Model file for the job. Use its own axes, mm. Face numbers are marked on the shaded views. A direction names the side the tool comes from. Round coordinates to 2 decimals unless told otherwise and drop trailing zeros. Loops run counter-clockwise (first coordinate to the right, second up) from the corner with the lowest first, then second, coordinate; pieces in that order, holes last. Notation, with made-up numbers: M -35.75,58 L 3.25,58 A16 cw 3.25,69 Z; hole C -25.5,24.5 d7. An arc over 180 degrees is marked long. Use a Markdown table: item, result. Add a question column.
Item 1: Wall check: L1, parallel to Y at x = 0.3, z = 15; L2, parallel to X at y = 50, z = 26.5; L3, parallel to Y at x = 11, z = 23.5. Give the ranges that are in metal, low to high. Write a range as from..to.
Item 2: Saw through at B-B on y = 40.5. Write the cut outline in (x, z).
Item 3: Pin check, flat tips, straight feed: P1, Ø2, axis at x = 1, y = 47, coming from the -Z side; P2, Ø12.5, axis at x = -11, z = 20.5, coming from the +Y side; P3, Ø9, axis at y = 36.5, z = 20.5, coming from the +X side; P4, Ø4, axis at x = -6.5, y = 9.5, coming from the +Z side. Stop position of each tip, or through.
Item 4: Saw through at D-D on y = 9. Write the cut outline in (x, z).
Item 5: Tool access for the marked faces 1 and 2: list every direction of +Z, -Z, +X, -X, +Y, -Y with a clear straight run to the whole face (end or side of a thin tool).
Item 6: Saw through at C-C on x = -0.5. Write the cut outline in (y, z).
Item 7: Two-plate mould, pull along Y, no slides. Class the marked faces 3, 4, 5 and 6: +Y half, -Y half, draft (parallel to the pull), parting line (faces both ways), or undercut.
Item 8: Saw through at A-A on z = 15. Write the cut outline in (x, y), then the cut area to 3 significant figures.
```python
from build123d import *

# Parameters (mm, degrees)
BOSS_EXTRUDE1_DEPTH = 30
SKETCH2_R           = 9.5
CUT_EXTRUDE1_DEPTH  = 70


with BuildPart() as part:
    # Sketch1 → Boss-Extrude1 (new body)
    with BuildSketch(Plane.XY):
        with BuildLine():
            Line((3.75, 0), (15, 0))
            Line((15, 0), (15, -4))
            Line((15, -4), (-15, -4))
            Line((-15, -4), (-15, 0))
            Line((-15, 0), (-3.75, 0))
            ThreePointArc((-3.75, 0), (-3.042893219, 0.292893219), (-2.75, 1))
            Line((-2.75, 1), (-2.75, 61))
            Line((-2.75, 61), (2.75, 61))
            Line((2.75, 61), (2.75, 1))
            ThreePointArc((2.75, 1), (3.042893219, 0.292893219), (3.75, 0))
        make_face()
    extrude(amount=BOSS_EXTRUDE1_DEPTH)

    # Sketch2 → Cut-Extrude1 (cut)
    with BuildSketch(Plane.ZY.offset(2.75)):
        with Locations((15, 40.5)):
            Circle(SKETCH2_R)
    extrude(amount=-CUT_EXTRUDE1_DEPTH, mode=Mode.SUBTRACT)


solid = part.part
```
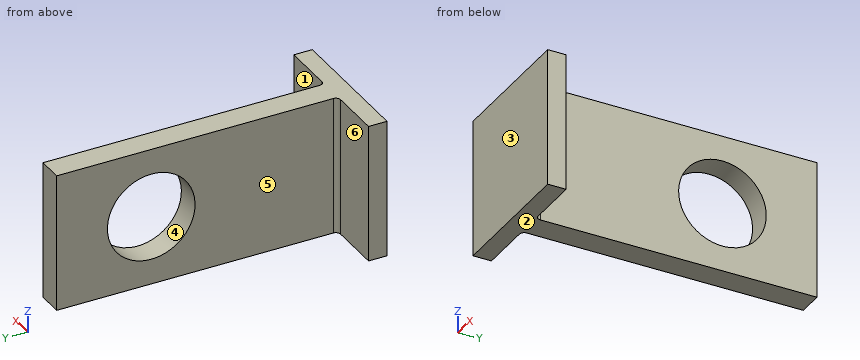
Entries:
| question | item | result |
|---|---|---|
| 1 | L1 | -4..31, 50..61 |
| 1 | L2 | -2.75..2.75 |
| 1 | L3 | -4..0 |
| 2 | outline | M -2.75,0 L 2.75,0 L 2.75,5.5 L -2.75,5.5 Z; M -2.75,24.5 L 2.75,24.5 L 2.75,30 L -2.75,30 Z |
| 3 | P1 | z = 0 |
| 3 | P2 | y = 0 |
| 3 | P3 | x = 2.75 |
| 3 | P4 | through |
| 4 | outline | M -2.75,0 L 2.75,0 L 2.75,30 L -2.75,30 Z |
| 5 | face 1 | +Z, -Z, +X, +Y |
| 5 | face 2 | -Z, +X, -X, +Y, -Y |
| 6 | outline | M -4,0 L 61,0 L 61,30 L -4,30 Z; hole C 40.5,15 d19 |
| 7 | face 3 | -Y half |
| 7 | face 4 | undercut |
| 7 | face 5 | draft |
| 7 | face 6 | +Y half |
| 8 | outline | M -15,-4 L 15,-4 L 15,0 L 3.75,0 A1 cw 2.75,1 L 2.75,31 L -2.75,31 L -2.75,1 A1 cw -3.75,0 L -15,0 Z; M -2.75,50 L 2.75,50 L 2.75,61 L -2.75,61 Z |
| 8 | area | 351 mm2 |
